from build123d import *

# Parameters (mm, degrees)
ESQUISSE3_R                  = 2.9
BOSS_EXTRU_1_DEPTH           = 1
ENL_V_MAT_EXTRU_1_DEPTH      = 8.7000001
ENL_V_MAT_EXTRU_1_DEPTH_BACK = 2
ESQUISSE7_W                  = 0.5
ESQUISSE7_H                  = 0.5


with BuildPart() as part:
    # Esquisse3 → Boss.-Extru.1 (new body)
    with BuildSketch(Plane.XY):
        Circle(ESQUISSE3_R)
    extrude(amount=BOSS_EXTRU_1_DEPTH)

    # Esquisse5 → Révolution1 (revolve)
    with BuildSketch(Plane(origin=(0, 0, 0), x_dir=(1, 0, 0), z_dir=(0, 1, 0))):
        with BuildLine():
            Line((0, -1), (0, -8.7))
            ThreePointArc((0, -8.7), (1.767766953, -7.96776677), (2.5, -6.199999817))
            Line((2.5, -6.199999817), (2.5, -1))
            Line((2.5, -1), (0, -1))
        make_face()
    revolve(axis=Axis((0, 0, 1), (0, 0, 1)))

    # Esquisse6 → Enlèv. mat.-Extru.1 (cut, two sides)
    with BuildSketch(Plane.XY.offset(1)) as enl_v_mat_extru_1_sk:
        Polygon((-2.5, 25.362745966), (-2.5, 1.469693846), (-2.5, -1.469693846), (-2.5, -25.362745966), (-50.286104241, -25.362745966), (-50.286104241, 25.362745966), align=None)
    extrude(amount=ENL_V_MAT_EXTRU_1_DEPTH, mode=Mode.SUBTRACT)
    extrude(enl_v_mat_extru_1_sk.sketch, amount=-ENL_V_MAT_EXTRU_1_DEPTH_BACK, mode=Mode.SUBTRACT)

    # Balayage1: sweep along a path in Esquisse8
    with BuildLine(Plane(origin=(0, 0, 0), x_dir=(0, 0, -1), z_dir=(1, 0, 0))) as balayage1_path:
        Line((0, 0), (1, 0))
        ThreePointArc((1, 0), (1.707106781, -0.292893219), (2, -1))
        Line((2, -1), (2, -5.5))
    # Esquisse7 → Balayage1 (sweep)
    with BuildSketch(Plane.XY):
        with Locations((1.27, 0)):
            Rectangle(ESQUISSE7_W, ESQUISSE7_H)
        with Locations((-1.27, 0)):
            Rectangle(ESQUISSE7_W, ESQUISSE7_H)
    sweep(path=balayage1_path.line)


solid = part.part
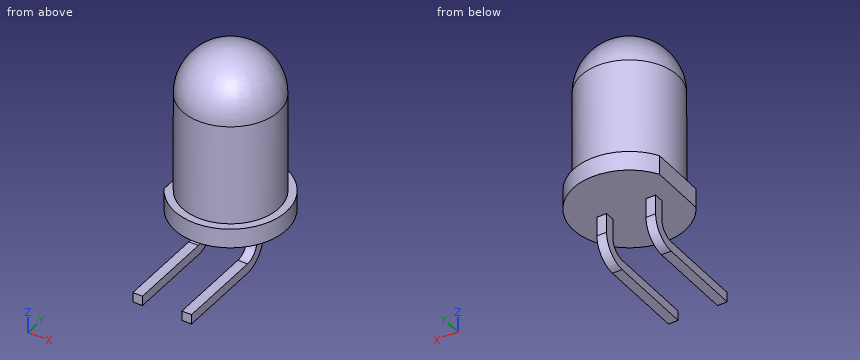
Check sheet for the modelled part. Datum: model origin and axes. Units: mm. Coordinates: 2 decimals unless noted, no trailing zeros. Loops run counter-clockwise (first coordinate to the right, second up) from the corner with the lowest first, then second, coordinate; pieces in that order, holes last. Notation, with made-up numbers: (-31.75, 81) -> (-5.75, 81) arc R32 ccw to (-5.75, 117) -> close; hole circle Ø4 at (-24.75, 37.25). An arc over 180 degrees is marked (long way). Answer in a Markdown table with one row per item.
1. Sectioned sample at B-B, the plane y = -3.75. Record the boundary of the cut face in (x, z), then the cut area to 3 significant figures.
Check values:
| item | result |
|---|---|
| outline | (-1.52, -2.25) -> (-1.02, -2.25) -> (-1.02, -1.75) -> (-1.52, -1.75) -> close; (1.02, -2.25) -> (1.52, -2.25) -> (1.52, -1.75) -> (1.02, -1.75) -> close |
| area | 0.500 mm2 |
2. Sectioned sample at D-D, the plane z = 5. Record the boundary of the cut face in (x, y).
Check values:
| item | result |
|---|---|
| outline | circle Ø5 at (0, 0) |
3. Sectioned sample at A-A, the plane z = -0.25. Record the boundary of the cut face in (x, y).
Check values:
| item | result |
|---|---|
| outline | (-1.52, -0.25) -> (-1.02, -0.25) -> (-1.02, 0.25) -> (-1.52, 0.25) -> close; (1.02, -0.25) -> (1.52, -0.25) -> (1.52, 0.25) -> (1.02, 0.25) -> close |
4. Material ranges on line 1 along Y through (x, z) = (-1.45, 7.25) (3 decimals); line 2 along Z through (x, y) = (-1.85, -1.25); line 3 along Y through (x, z) = (-0.15, 1.5), recorded low to high. Write a range as [from, to].
Check values:
| item | result |
|---|---|
| line 1 | y = [-1.745, 1.745] |
| line 2 | z = [0, 7.32] |
| line 3 | y = [-2.5, 2.5] |
5. Go/stop test with flat-tipped pins: pin 1 (1.8 mm diameter, centred on y = -1.5, z = -1.5, fed in from -X); pin 2 (3 mm diameter, centred on x = -1, y = -1.5, fed in from -Z); pin 3 (2 mm diameter, centred on y = -2.5, z = 5, fed in from -X); pin 4 (1.8 mm diameter, centred on y = -1.5, z = -1.5, fed in from +X). Record where each tip stops, or that it passes through.
Check values:
| item | result |
|---|---|
| pin 1 | stops at x = -1.52 |
| pin 2 | stops at z = -2.25 |
| pin 3 | stops at x = -2 |
| pin 4 | stops at x = 1.52 |
6. Sectioned sample at C-C, the plane y = -0.5. Give the number of separate pieces and of enclosed holes in the cut face, then the cut area to 3 significant figures.
Check values:
| item | result |
|---|---|
| separate pieces | 3 |
| enclosed holes | 0 |
| area | 40.8 mm2 |
